Design review of the part built by this model. Coordinates are the model's own, in mm. A direction names the side the tool comes from. Coordinates: 2 decimals unless noted, no trailing zeros. Answer as a JSON object with one key per item and string values.
Autodesk Inventor part; units mm, degrees
ref_plane "YZ Plane" through (0, 0, 0) normal (1, 0, 0) x (0, 1, 0)
ref_plane "XZ Plane" through (0, 0, 0) normal (0, 1, 0) x (-1, 0, 0)
ref_plane "XY Plane" through (0, 0, 0) normal (0, 0, 1) x (1, 0, 0)
sketch "Sketch1" plane through (0, 0, 0) normal (0, 0, 1) x (1, 0, 0)
  circle A0 centre (0, 0) radius 33.02
  circle A1 centre (0, 0) radius 36.068
  dimension "d0" = 66.04
  dimension "d1" = 72.136
extrude "Extrusion1" add sketch "Sketch1" along normal blind 37.592
sketch "Sketch2" plane through (0, 0, 37.592) normal (0, 0, 1) x (1, 0, 0)
  circle A0 centre (0, 0) radius 36.068
  circle A1 centre (0, 0) radius 36.068
extrude "Extrusion2" add sketch "Sketch2" along normal blind 8.2804
sketch "Sketch3" plane through (0, 0, 45.8724) normal (0, 0, 1) x (1, 0, 0)
  circle A0 centre (0, 0) radius 36.068
  circle A1 centre (0, 0) radius 10.4648
  circle A2 centre (0, 0) radius 1.905
  dimension "d6" = 20.9296
  dimension "d7" = 3.81
extrude "Extrusion3" add sketch "Sketch3" along normal blind 7.874 contours A1
sketch "Sketch4" plane through (0, 0, 45.8724) normal (0, 0, 1) x (1, 0, 0)
  circle A0 centre (0, 0) radius 36.068
  circle A1 centre (0, 0) radius 10.4648
  circle A2 centre (0, 0) radius 36.068
  circle A3 centre (0, 0) radius 33.02
  dimension "d10" = 66.04
extrude "Extrusion4" add sketch "Sketch4" along normal blind 33.3756 contours A0
sketch "Sketch5" plane through (0, 0, 37.592) normal (0, 0, -1) x (-1, 0, 0)
  circle A0 centre (0, 0) radius 33.02
  line L0 (2.1997, -3.81) -> (-2.1997, -3.81)
  line L1 (-2.1997, -3.81) -> (-4.3994, 0)
  line L2 (-4.3994, 0) -> (-2.1997, 3.81)
  line L3 (-2.1997, 3.81) -> (2.1997, 3.81)
  line L4 (2.1997, 3.81) -> (4.3994, 0)
  line L5 (4.3994, 0) -> (2.1997, -3.81)
  dimension "d13" = 7.62
extrude "Extrusion5" cut sketch "Sketch5" against normal blind 10.414 contours L0 L1 L2 L3 L4 L5
sketch "Sketch6" plane through (0, 0, 37.592) normal (0, 0, -1) x (-1, 0, 0)
  circle A0 centre (0, 0) radius 33.02
  circle A1 centre (0, 0) radius 16.891
  circle A2 centre (0, 0) radius 33.02
  line L0 (0.635, 33.0139) -> (0.635, 18.1499)
  line L1 (-0.635, 18.1499) -> (-0.635, 33.0139)
  line L2 (-28.9084, -15.957) -> (-16.0358, -8.525)
  line L3 (-15.4008, -9.6249) -> (-28.2734, -17.0569)
  line L4 (28.2734, -17.0569) -> (15.4008, -9.6249)
  line L5 (16.0358, -8.525) -> (28.9084, -15.957)
  arc A3 (-0.635, 18.1499) -> (-16.0358, -8.525) centre (0, 0) ccw
  arc A4 (-15.4008, -9.6249) -> (15.4008, -9.6249) centre (0, 0) ccw
  arc A5 (16.0358, -8.525) -> (0.635, 18.1499) centre (0, 0) ccw
  arc A6 (0.635, 33.0139) -> (-0.635, 33.0139) centre (0, 0) ccw
  arc A7 (-28.9084, -15.957) -> (-28.2734, -17.0569) centre (0, 0) ccw
  arc A8 (28.2734, -17.0569) -> (28.9084, -15.957) centre (0, 0) ccw
  dimension "d16" = 33.782
  dimension "d18" = 1.27
  dimension "d19" = 0.635
  dimension "d22" = 360
extrude "Extrusion6" add sketch "Sketch6" along normal blind 8.128 contours L0 A5 L5 A0 L4 A4 L3 L2 A3 L1
sketch "Sketch7" plane through (0, 0, 0) normal (1, 0, 0) x (0, 1, 0)
  line L0 (-10.4648, 45.8724) -> (-10.4648, 53.7464)
  line L1 (-10.4648, 53.7464) -> (-1.905, 53.7464)
  line L2 (-1.905, 53.7464) -> (-1.905, 48.006)
  line L3 (-1.905, 48.006) -> (-3.81, 48.006)
  line L4 (-3.81, 48.006) -> (-3.81, 37.592)
  line L5 (-3.81, 37.592) -> (-16.891, 37.592)
  line L6 (-16.891, 37.592) -> (-16.891, 29.464)
  line L7 (-16.891, 29.464) -> (-18.161, 29.464)
  line L8 (-18.161, 29.464) -> (-18.161, 37.592)
  line L9 (-18.161, 37.592) -> (-33.02, 37.592)
  line L10 (-33.02, 37.592) -> (-33.02, 0)
  line L11 (-33.02, 0) -> (-36.068, 0)
  line L12 (-36.068, 0) -> (-36.068, 79.248)
  line L13 (-36.068, 79.248) -> (-33.02, 79.248)
  line L14 (-33.02, 79.248) -> (-33.02, 45.8724)
  line L15 (-33.02, 45.8724) -> (-10.4648, 45.8724)
  line L16 (10.4648, 53.7464) -> (10.4648, 45.8724)
  line L17 (10.4648, 45.8724) -> (33.02, 45.8724)
  line L18 (33.02, 45.8724) -> (33.02, 79.248)
  line L19 (33.02, 79.248) -> (36.068, 79.248)
  line L20 (36.068, 79.248) -> (36.068, 0)
  line L21 (36.068, 0) -> (33.02, 0)
  line L22 (33.02, 0) -> (33.02, 29.464)
  line L23 (33.02, 29.464) -> (16.891, 29.464)
  line L24 (16.891, 29.464) -> (16.891, 37.592)
  line L25 (16.891, 37.592) -> (3.81, 37.592)
  line L26 (3.81, 37.592) -> (3.81, 48.006)
  line L27 (3.81, 48.006) -> (1.905, 48.006)
  line L28 (1.905, 48.006) -> (1.905, 53.7464)
  line L29 (1.905, 53.7464) -> (10.4648, 53.7464)
  line L30 (36.068, 79.248) -> (36.068, 0)
  line L31 (-36.068, 79.248) -> (36.068, 79.248)
  line L32 (-36.068, 0) -> (36.068, 0)
  line L33 (36.068, 79.248) -> (42.672, 79.248)
  line L34 (36.068, 0) -> (42.672, 0)
  line L35 (0, 98.0875) -> (0, -23.6959) construction
  line L36 (-10.4648, 45.8724) -> (-10.4648, 53.7464) construction
  line L37 (-10.4648, 53.7464) -> (-1.905, 53.7464) construction
  line L38 (-1.905, 53.7464) -> (-1.905, 48.006) construction
  line L39 (-1.905, 48.006) -> (-3.81, 48.006) construction
  line L40 (-3.81, 37.592) -> (-16.891, 37.592) construction
  line L41 (-16.891, 37.592) -> (-16.891, 29.464) construction
  line L42 (-16.891, 29.464) -> (-18.161, 29.464) construction
  line L43 (-18.161, 29.464) -> (-18.161, 37.592) construction
  line L44 (-18.161, 37.592) -> (-33.02, 37.592) construction
  line L45 (-33.02, 37.592) -> (-33.02, 0) construction
  line L46 (-33.02, 0) -> (-36.068, 0) construction
  line L47 (-36.068, 0) -> (-36.068, 79.248) construction
  line L48 (-36.068, 79.248) -> (-33.02, 79.248) construction
  line L49 (-33.02, 79.248) -> (-33.02, 45.8724) construction
  line L50 (-33.02, 45.8724) -> (-10.4648, 45.8724) construction
  line L51 (10.4648, 53.7464) -> (10.4648, 45.8724) construction
  line L52 (10.4648, 45.8724) -> (33.02, 45.8724) construction
  line L53 (33.02, 45.8724) -> (33.02, 79.248) construction
  line L54 (33.02, 79.248) -> (36.068, 79.248) construction
  line L55 (36.068, 79.248) -> (36.068, 0) construction
  line L56 (36.068, 0) -> (33.02, 0) construction
  line L57 (33.02, 0) -> (33.02, 29.464) construction
  line L58 (33.02, 29.464) -> (16.891, 29.464) construction
  line L59 (16.891, 29.464) -> (16.891, 37.592) construction
  line L60 (16.891, 37.592) -> (3.81, 37.592) construction
  line L61 (3.81, 48.006) -> (1.905, 48.006) construction
  line L62 (1.905, 48.006) -> (1.905, 53.7464) construction
  line L63 (1.905, 53.7464) -> (10.4648, 53.7464) construction
  line L64 (-10.4648, 45.8724) -> (-10.4648, 53.7464) construction
  line L65 (-10.4648, 53.7464) -> (-1.905, 53.7464) construction
  line L66 (-1.905, 53.7464) -> (-1.905, 48.006) construction
  line L67 (-1.905, 48.006) -> (-3.81, 48.006) construction
  line L68 (-3.81, 37.592) -> (-16.891, 37.592) construction
  line L69 (-16.891, 37.592) -> (-16.891, 29.464) construction
  line L70 (-16.891, 29.464) -> (-18.161, 29.464) construction
  line L71 (-18.161, 29.464) -> (-18.161, 37.592) construction
  line L72 (-18.161, 37.592) -> (-33.02, 37.592) construction
  line L73 (-33.02, 37.592) -> (-33.02, 0) construction
  line L74 (-33.02, 0) -> (-36.068, 0) construction
  line L75 (-36.068, 0) -> (-36.068, 79.248) construction
  line L76 (-36.068, 79.248) -> (-33.02, 79.248) construction
  line L77 (-33.02, 79.248) -> (-33.02, 45.8724) construction
  line L78 (-33.02, 45.8724) -> (-10.4648, 45.8724) construction
  line L79 (10.4648, 53.7464) -> (10.4648, 45.8724) construction
  line L80 (10.4648, 45.8724) -> (33.02, 45.8724) construction
  line L81 (33.02, 45.8724) -> (33.02, 79.248) construction
  line L82 (33.02, 79.248) -> (36.068, 79.248) construction
  line L83 (36.068, 79.248) -> (36.068, 0) construction
  line L84 (36.068, 0) -> (33.02, 0) construction
  line L85 (33.02, 0) -> (33.02, 29.464) construction
  line L86 (33.02, 29.464) -> (16.891, 29.464) construction
  line L87 (16.891, 29.464) -> (16.891, 37.592) construction
  line L88 (16.891, 37.592) -> (3.81, 37.592) construction
  line L89 (3.81, 48.006) -> (1.905, 48.006) construction
  line L90 (1.905, 48.006) -> (1.905, 53.7464) construction
  line L91 (1.905, 53.7464) -> (10.4648, 53.7464) construction
  line L92 (-36.068, 79.248) -> (-36.068, 0)
  line L93 (-36.068, 79.248) -> (-42.672, 79.248)
  line L94 (-36.068, 0) -> (-42.672, 0)
  ellipse E0 centre (45.4728, 39.624) end of major axis (27.4456, 39.624) minor radius 40.1111 (42.672, 0) -> (42.672, 79.248) ccw
  ellipse E1 centre (-45.4728, 39.624) end of major axis (-27.4456, 39.624) minor radius 40.1111 (-42.672, 79.248) -> (-42.672, 0) ccw
  line L95 (-63.5, 14.7973) -> (-63.5, 63.5963) construction
  line L96 (63.5, 9.0713) -> (63.5, 59.5395) construction
  line L97 (-3.81, 48.006) -> (-3.81, 37.592)
  line L98 (3.81, 37.592) -> (3.81, 48.006)
  line L99 (-3.81, 48.006) -> (-3.81, 37.592)
  line L100 (3.81, 37.592) -> (3.81, 48.006)
  point P0 (0, 0)
  dimension "d26" = 6.604
  dimension "d27" = 6.604
  dimension "d31" = 127
revolve "Revolution1" add sketch "Sketch7" angle 360 about axis through (0, 0, 98.0875) along (0, 0, -1) contours L12 L94 E1 L93 | L33 E0 L34 L20
sketch "Sketch8" plane through (0, 0, 45.8724) normal (0, 0, 1) x (1, 0, 0)
  circle A0 centre (0, 0) radius 33.02
  circle A1 centre (0, 16.7005) radius 4.7625
  circle A2 centre (0, 0) radius 1.905 construction
  line L0 (0, 0) -> (0, 23.6357) construction
  circle A3 centre (-11.809, 11.809) radius 4.7625
  circle A4 centre (-16.7005, 0) radius 4.7625
  circle A5 centre (-11.809, -11.809) radius 4.7625
  circle A6 centre (0, -16.7005) radius 4.7625
  circle A7 centre (11.809, -11.809) radius 4.7625
  circle A8 centre (16.7005, 0) radius 4.7625
  circle A9 centre (11.809, 11.809) radius 4.7625
  dimension "d33" = 9.525
  dimension "d34" = 16.7005
  dimension "d37" = 360
extrude "Extrusion7" cut sketch "Sketch8" against normal blind 5.334 contours A1 | A3 | A4 | A5 | A6 | A7 | A8 | A9
properties part number "Large Wheel"
1) Tool access review of faces 1 (the cylindrical face through (-0.41, 1.86, 50.84)), 2 (the flat face through (3.315, 1.878, 42.726)), 3 (the cylindrical face through (-2.269, 10.216, 49.754)): name each direction out of +Z, -Z, +X, -X, +Y, -Y from which nothing blocks a thin tool from reaching the whole face with its end or side.
Taken from the geometry:
{"face 1": "+Z, -Z", "face 2": "-Z", "face 3": "+Z"}
2) Add section A-A (z = 35). Count the separate pieces of the cut face and the enclosed holes in it, and give its area (3 significant figures).
Taken from the geometry:
{"separate pieces": "1", "enclosed holes": "4", "area": "9,390 mm2"}
3) To check wall thickness, follow L1, parallel to X at y = -13, z = 41; L2, parallel to Z at x = 36, y = -0.5; L3, parallel to Y at x = -21.5, z = 57. State the ranges of each line that lie inside material, in increasing order.
Taken from the geometry:
{"L1": "x = -62.14 to -16.42, -7.2 to -3, 3 to 7.2, 16.42 to 62.14", "L2": "z = 0 to 79.25", "L3": "y = -57.85 to -25.06, 25.06 to 57.85"}
4) Insertion check: pin 1 Ø2 at (x, z) = (-1, 42.5) entering from +Y; pin 2 Ø5 at (x, y) = (2, -16) entering from +Z; pin 3 Ø7.5 at (x, y) = (-2.5, 19) entering from +Z. Each pin has a flat end and moves straight along its axis. Give the tip position at first contact, or say it passes through.
Taken from the geometry:
{"pin 1": "stops at y = 63.48", "pin 2": "stops at z = 40.54", "pin 3": "stops at z = 45.87"}
